from build123d import *

# Parameters (mm, degrees)
SKETCH_R  = 1.8288
PAD_DEPTH = 3


with BuildPart() as part:
    # Sketch → Pad (new body)
    with BuildSketch(Plane.XY):
        with BuildLine():
            ThreePointArc((-154.4, 333.375), (-155.107107, 333.082107), (-155.4, 332.375))
            Line((-155.4, 1), (-155.4, 332.375))
            ThreePointArc((-155.4, 1), (-155.107107, 0.292893), (-154.4, 0))
            Line((-154.4, 0), (-89.852, 0))
            ThreePointArc((-89.852, 0), (-89.144893, 0.292893), (-88.852, 1))
            Line((-88.852, 12.7), (-88.852, 1))
            ThreePointArc((-82.248, 12.7), (-85.55, 16.002), (-88.852, 12.7))
            Line((-82.248, 12.7), (-82.248, 1))
            ThreePointArc((-82.248, 1), (-81.955107, 0.292893), (-81.248, 0))
            Line((-81.248, 0), (15.248, 0))
            ThreePointArc((15.248, 0), (15.955107, 0.292893), (16.248, 1))
            Line((16.248, 12.7), (16.248, 1))
            ThreePointArc((22.852, 12.7), (19.55, 16.002), (16.248, 12.7))
            Line((22.852, 12.7), (22.852, 1))
            ThreePointArc((22.852, 1), (23.144893, 0.292893), (23.852, 0))
            Line((23.852, 0), (37.6, 0))
            ThreePointArc((37.6, 0), (38.307107, 0.292893), (38.6, 1))
            Line((38.6, 1), (38.6, 24.9))
            ThreePointArc((39.6, 25.9), (38.892893, 25.607107), (38.6, 24.9))
            Line((39.6, 25.9), (154.4, 25.9))
            ThreePointArc((154.4, 25.9), (155.107107, 26.192893), (155.4, 26.9))
            Line((155.4, 332.375), (155.4, 26.9))
            ThreePointArc((155.4, 332.375), (155.107107, 333.082107), (154.4, 333.375))
            Line((-154.4, 333.375), (154.4, 333.375))
        make_face()
        with Locations((-141.9352, 327.025)):
            Circle(SKETCH_R, mode=Mode.SUBTRACT)
        with Locations((-141.9352, 166.6875)):
            Circle(SKETCH_R, mode=Mode.SUBTRACT)
        with Locations((141.9352, 327.025)):
            Circle(SKETCH_R, mode=Mode.SUBTRACT)
        with Locations((141.9352, 166.6875)):
            Circle(SKETCH_R, mode=Mode.SUBTRACT)
    extrude(amount=PAD_DEPTH)


solid = part.part
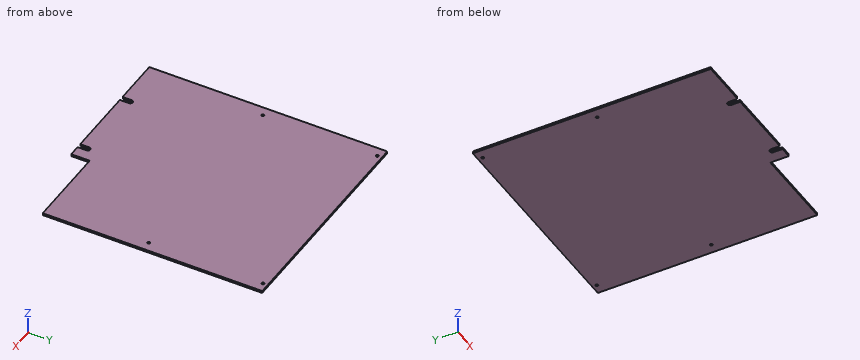
Geometry check sheet. Reference: the model listing, model coordinates, mm. Coordinates: 2 decimals unless noted, no trailing zeros. Order: outer loops, then holes, each group sorted by start corner. A loop starts at its lowest first (then second) coordinate and runs counter-clockwise, first axis right, second up. Notation, with made-up numbers: (40.25, 54) -> (44.25, 54) arc R11 ccw to (44.25, 61) -> close; hole circle Ø3 at (-27, 42). An arc over 180 degrees is marked (long way). Use a Markdown table: item, result. Add a question column.
1. Material ranges on L1, parallel to Y at x = 107, z = 1.25 (3 decimals); L2, parallel to Y at x = -86, z = 1.45 (3 decimals); L3, parallel to X at y = 25, z = 1.9, recorded low to high.
2. Go/stop test with flat-tipped pins: pin 1 Ø1.5 at (x, z) = (114, 1.5) entering from -Y; pin 2 Ø1.5 at (x, y) = (36.5, 75) entering from -Z; pin 3 Ø0.9 at (y, z) = (4.5, 1.5) entering from +X. Record where each tip stops, or that it passes through.
3. Cross-section at A-A (z = 1.8). Give the number of separate pieces and of enclosed holes in the cut face, and give its area (3 significant figures).
4. Cross-section at B-B (x = 136). Enter the section's corners in (y, z) (3 decimals).
Filled sheet:
| question | item | result |
|---|---|---|
| 1 | L1 | 25.9 to 333.375 |
| 1 | L2 | 15.971 to 333.375 |
| 1 | L3 | -155.4 to 38.61 |
| 2 | pin 1 | y = 25.9 |
| 2 | pin 2 | z = 0 |
| 2 | pin 3 | x = 38.6 |
| 3 | separate pieces | 1 |
| 3 | enclosed holes | 4 |
| 3 | area | 100,000 mm2 |
| 4 | outline | (25.9, 0) -> (333.375, 0) -> (333.375, 3) -> (25.9, 3) -> close |
